from build123d import *

# Parameters (mm, degrees)
BOSS_EXTRUDE1_DEPTH = 80
SKETCH3_R           = 3.5
CUT_EXTRUDE1_DEPTH  = 25
CUT_EXTRUDE2_REACH  = 27
SKETCH4_R           = 3


with BuildPart() as part:
    # Sketch2 → Boss-Extrude1 (new body)
    with BuildSketch(Plane.XY):
        Polygon((23, 25), (25, 25), (25, 0), (0, 0), (0, 25), (2, 25), (2, 2), (23, 2), align=None)
    extrude(amount=BOSS_EXTRUDE1_DEPTH)

    # Sketch3 → Cut-Extrude1 (cut)
    with BuildSketch(Plane(origin=(25, 0, 0), x_dir=(0, 0, -1), z_dir=(1, 0, 0))):
        with Locations((-65, 12.5)):
            Circle(SKETCH3_R)
    extrude(amount=-CUT_EXTRUDE1_DEPTH, mode=Mode.SUBTRACT)

    # Sketch4 → Cut-Extrude2 (cut, up to next)
    with BuildSketch(Plane.XZ, mode=Mode.PRIVATE) as cut_extrude2_sk1:
        with Locations((12.5, 60)):
            Circle(SKETCH4_R)
    cut_extrude2_tool1 = extrude(cut_extrude2_sk1.sketch, amount=-CUT_EXTRUDE2_REACH, mode=Mode.PRIVATE) & part.part
    add(cut_extrude2_tool1.solids().sort_by_distance((12.5, 0, 60))[0], mode=Mode.SUBTRACT)
    # Sketch4 → Cut-Extrude2 (cut, up to next)
    with BuildSketch(Plane.XZ, mode=Mode.PRIVATE) as cut_extrude2_sk2:
        with Locations((12.5, 20)):
            Circle(SKETCH4_R)
    cut_extrude2_tool2 = extrude(cut_extrude2_sk2.sketch, amount=-CUT_EXTRUDE2_REACH, mode=Mode.PRIVATE) & part.part
    add(cut_extrude2_tool2.solids().sort_by_distance((12.5, 0, 20))[0], mode=Mode.SUBTRACT)


solid = part.part
Can you work these out from the model? Positions are in its coordinate system, mm. A direction names the side the tool comes from. Give positions to 0.01 mm unless a question says otherwise; leave off trailing zeros. Loops run counter-clockwise (first coordinate to the right, second up) from the corner with the lowest first, then second, coordinate; pieces in that order, holes last. Notation, with made-up numbers: (80, 74.25) - (112, 74.25) arc R16 cw to (112, 89.25) - close; hole circle Ø2 at (-7.5, 81). An arc over 180 degrees is marked (long way). Return JSON: item names as keys, results as strings.
1. I want a section at B-B on z = 20. Please give me the cut outline in (x, y).
Output values:
{"outline": "(0, 0) - (9.5, 0) - (9.5, 2) - (2, 2) - (2, 25) - (0, 25) - close; (15.5, 0) - (25, 0) - (25, 25) - (23, 25) - (23, 2) - (15.5, 2) - close"}
2. I want a section at C-C on y = 12.5. Please give me the cut outline in (x, z).
Output values:
{"outline": "(0, 0) - (2, 0) - (2, 61.5) - (0, 61.5) - close; (0, 68.5) - (2, 68.5) - (2, 80) - (0, 80) - close; (23, 0) - (25, 0) - (25, 61.5) - (23, 61.5) - close; (23, 68.5) - (25, 68.5) - (25, 80) - (23, 80) - close"}
3. I want a section at A-A on x = 12.5. Please give me the cut outline in (y, z).
Output values:
{"outline": "(0, 0) - (2, 0) - (2, 17) - (0, 17) - close; (0, 23) - (2, 23) - (2, 57) - (0, 57) - close; (0, 63) - (2, 63) - (2, 80) - (0, 80) - close"}
4. I want a section at D-D on z = 65. Please give me the cut outline in (x, y).
Output values:
{"outline": "(0, 0) - (25, 0) - (25, 9) - (23, 9) - (23, 2) - (2, 2) - (2, 9) - (0, 9) - close; (0, 16) - (2, 16) - (2, 25) - (0, 25) - close; (23, 16) - (25, 16) - (25, 25) - (23, 25) - close"}
5. We'd pull the mould along Z, two halves only. Please class faces 3 (the face through (23, 13, 39)), 4 (the face through (13, 1, 80)), 5 (the face through (1, 10.4, 67.8)): +Z half, -Z half, draft (parallel to the pull), parting line (faces both ways), or undercut.
Output values:
{"face 3": "draft", "face 4": "+Z half", "face 5": "undercut"}
6. For faces 1 (the face through (25, 13, 39)), 2 (the face through (12, 2, 39)), which set-ups out of +Z, -Z, +X, -X, +Y, -Y let a thin tool reach every point of the face, with its end or its side?
Output values:
{"face 1": "+Z, -Z, +X, +Y, -Y", "face 2": "+Z, -Z, +Y"}
7. If I drill on line 1 (Z direction, x = 12.5, y = 0.75); line 2 (X direction, y = 4, z = 27.5); line 3 (Y direction, x = 0.5, z = 65), over which ranges is the centre line in solid material (lowest first)?
Output values:
{"line 1": "z = 0 to 17, 23 to 57, 63 to 80", "line 2": "x = 0 to 2, 23 to 25", "line 3": "y = 0 to 9, 16 to 25"}
8. I'm going to push flat-ended pins straight in: pin 1 Ø5.5 at (x, z) = (12.5, 20) entering from -Y; pin 2 Ø6.5 at (x, z) = (11.5, 58) entering from +Y; pin 3 Ø5 at (x, z) = (15.5, 59) entering from -Y. Where does each tip first touch, or does it pass through?
Output values:
{"pin 1": "passes through", "pin 2": "stops at y = 2", "pin 3": "stops at y = 0"}
